Autodesk Inventor part; units mm, degrees
ref_plane "YZ Plane" through (0, 0, 0) normal (1, 0, 0) x (0, 1, 0)
ref_plane "XZ Plane" through (0, 0, 0) normal (0, 1, 0) x (-1, 0, 0)
ref_plane "XY Plane" through (0, 0, 0) normal (0, 0, 1) x (1, 0, 0)
sketch "Sketch1" plane through (0, 0, 0) normal (0, 0, 1) x (1, 0, 0)
  line L0 (0, 17) -> (12, 17)
  line L1 (12, 17) -> (12, 11)
  line L2 (12, 11) -> (0, 11)
  line L3 (0, 11) -> (0, 17)
  line L4 (0, 6) -> (12, 6)
  line L5 (12, 6) -> (12, 0)
  line L6 (12, 0) -> (0, 0)
  line L7 (0, 0) -> (0, 6)
  dimension "d0" = 6
  dimension "d1" = 5
  dimension "d2" = 12
extrude "Extrusion1" add sketch "Sketch1" along normal blind 3 contours L4 L5 L6 L7
sketch "Sketch2" plane through (0, 0, 3) normal (0, 0, 1) x (1, 0, 0)
  line L0 (16.7529, 15.7773) -> (28.7529, 15.7773)
  line L1 (28.7529, 22.7773) -> (22.7529, 22.7773)
  line L2 (22.7529, 22.7773) -> (22.7529, 15.7773)
  line L3 (22.7529, 15.7773) -> (28.7529, 15.7773)
  line L4 (28.7529, 15.7773) -> (28.7529, 22.7773)
  line L5 (28.7529, 22.7773) -> (16.7529, 22.7773)
  line L6 (28.7529, 15.7773) -> (28.7529, 22.7773)
  line L7 (12, 6) -> (6, 6)
  line L8 (6, 6) -> (6, 0)
  line L9 (6, 0) -> (12, 0)
  line L10 (12, 0) -> (12, 6)
  line L11 (0, 0) -> (12, 0)
  dimension "d5" = 6
extrude "Extrusion2" add sketch "Sketch2" along normal blind 20 contours L10 L9 L8 L7
sketch "Sketch3" plane through (0, 6, 0) normal (0, 1, 0) x (1, 0, 0)
  circle A0 centre (9, -20) radius 2
  line L0 (12, -23) -> (6, -23)
  line L1 (12, 0) -> (12, -23)
  point P0 (-16.7529, 0)
  dimension "d8" = 3
  dimension "d9" = 3
  dimension "d10" = 4
extrude "Extrusion3" cut sketch "Sketch3" against normal blind 30
chamfer "Chamfer1" distance 2 angle 45 2 edges at (12, 3, 0) (0, 3, 0)
sketch "Sketch4" plane through (12, 0, 23) normal (1, 0, 0) x (0, 0, -1)
  line L0 (8, 11.5882) -> (10, 11.5882)
  line L1 (10, 11.5882) -> (10, -21.6618)
  line L2 (10, -21.6618) -> (8, -21.6618)
  line L3 (8, -21.6618) -> (8, 11.5882)
  line L4 (0, 0) -> (0, 7)
  point P0 (23, -15.7773)
  dimension "d16" = 2
  dimension "d17" = 8
extrude "Extrusion4" cut sketch "Sketch4" against normal blind 1
properties part number "arms01"
Could you check a few things on this model? Use its own coordinates, in mm. A direction names the side the tool comes from. Coordinates: 2 decimals unless noted, no trailing zeros. Order: outer loops, then holes, each group sorted by start corner. A loop starts at its lowest first (then second) coordinate and runs counter-clockwise, first axis right, second up. Notation, with made-up numbers: (4.5, 7) - (39.5, 7) arc R36 ccw to (39.5, 45) - close; hole circle Ø2 at (41.5, 14). An arc over 180 degrees is marked (long way). Answer in a Markdown table with one row per item. Add a question column.
(1) On a 3-axis mill with a long thin cutter (end or side, diameter ignored), from which of +Z, -Z, +X, -X, +Y, -Y can I reach the whole of each face in a straight line? I mean faces 1 (the face through (6, 3, 13)), 2 (the face through (9, 0, 9)), 3 (the face through (11.5, 3, 15)). Say none if no direction works.
(2) If we section it at C-C, the plane y = 1.3: Please give me the cut outline in (x, z).
(3) If we section it at A-A, the plane z = 20: Please give me the cut outline in (x, y), then the cut area to 3 significant figures.
(4) Will these pins go through, and if not, where does the flat tip stop? pin 1 (3 mm diameter, centred on x = 3.5, y = 3.5, fed in from +Z); pin 2 (1.8 mm diameter, centred on y = 3, z = 9, fed in from -X); pin 3 (0.5 mm diameter, centred on x = 11.5, y = 2, fed in from -Z).
(5) If we section it at B-B, the plane x = 9: Please give me the cut outline in (y, z), then the cut area to 3 significant figures.
(6) If we section it at D-D, the plane z = 5.25: Please give me the cut outline in (x, y).
(7) I need wall thicknesses on L1, parallel to Z at x = 9, y = 2.35; L2, parallel to X at y = 1.8, z = 20; L3, parallel to Z at x = 9.5, y = 2.75. Which ranges of each line are inside material? Lowest first, please.
(8) If we mould it in two halves opening along Z, with no side actions, what happens to faces 4 (the face through (11.5, 3, 13)), 5 (the face through (0, 3, 2.5)), 6 (the face through (6, 3, 0)), 7 (the face through (3, 3, 3))? For each: released by +Z, released by -Z, zero draft, split by the parting line, or undercut.
Results are:
| question | item | result |
|---|---|---|
| 1 | face 1 | +Z, -X, +Y, -Y |
| 1 | face 2 | +Z, -Z, +X, -X, -Y |
| 1 | face 3 | +X, +Y, -Y |
| 2 | outline | (0, 2) - (2, 0) - (10, 0) - (12, 2) - (12, 13) - (11, 13) - (11, 15) - (12, 15) - (12, 23) - (6, 23) - (6, 3) - (0, 3) - close; hole circle Ø4 at (9, 20) |
| 3 | outline | (6, 0) - (7, 0) - (7, 6) - (6, 6) - close; (11, 0) - (12, 0) - (12, 6) - (11, 6) - close |
| 3 | area | 12.0 mm2 |
| 4 | pin 1 | stops at z = 3 |
| 4 | pin 2 | stops at x = 6 |
| 4 | pin 3 | stops at z = 1.25 |
| 5 | outline | (0, 0) - (6, 0) - (6, 18) - (0, 18) - close; (0, 22) - (6, 22) - (6, 23) - (0, 23) - close |
| 5 | area | 114 mm2 |
| 6 | outline | (6, 0) - (12, 0) - (12, 6) - (6, 6) - close |
| 7 | L1 | z = 0 to 18, 22 to 23 |
| 7 | L2 | x = 6 to 7, 11 to 12 |
| 7 | L3 | z = 0 to 18.06, 21.94 to 23 |
| 8 | face 4 | undercut |
| 8 | face 5 | zero draft |
| 8 | face 6 | released by -Z |
| 8 | face 7 | released by +Z |
